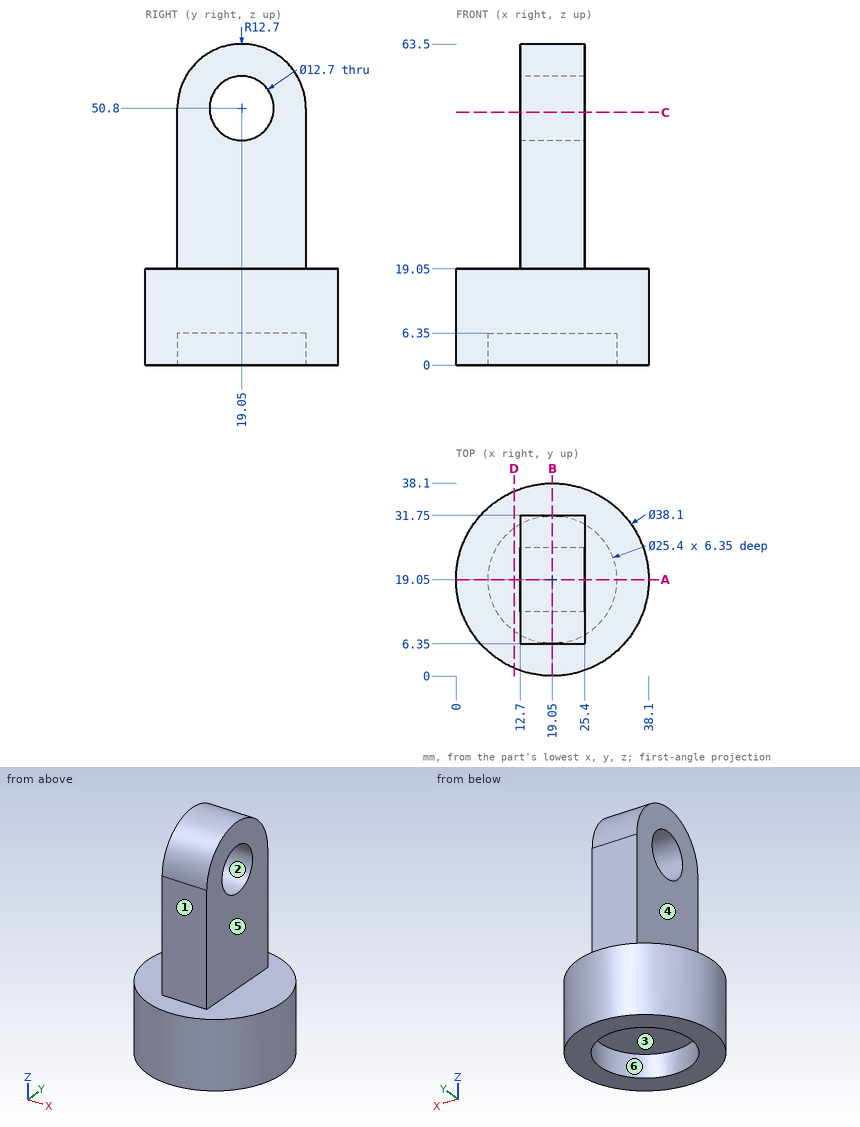
Can you work these out from the drawing? Everything is in mm from the part's minimum corner. A direction names the side the tool comes from. Round coordinates to 2 decimals unless told otherwise and drop trailing zeros. Loops run counter-clockwise (first coordinate to the right, second up) from the corner with the lowest first, then second, coordinate; pieces in that order, holes last. Notation, with made-up numbers: (18.5, -15.75) -> (67.5, -15.75) arc R15 ccw to (67.5, 10.25) -> close; hole circle Ø3 at (45.5, 76). An arc over 180 degrees is marked (long way). One line per question, with ' | ' between items.
(1) If we section it at D-D on x = 11.5: List the corners of the cut face in (y, z) for me.
Model answer:
outline: (1.56, 0) -> (8.84, 0) -> (8.84, 6.35) -> (29.26, 6.35) -> (29.26, 0) -> (36.54, 0) -> (36.54, 19.05) -> (1.56, 19.05) -> close
(2) If I drill on probe 1 along Y at (x, z) = (19.05, 4); probe 2 along Z at (x, y) = (34.5, 30), over which ranges is the centre line in solid material (lowest first)?
Model answer:
probe 1: y = 0 to 6.35, 31.75 to 38.1 | probe 2: z = 0 to 19.05
(3) If we section it at B-B on x = 19.05: List the corners of the cut face in (y, z) for me, and give its area (3 significant figures).
Model answer:
outline: (0, 0) -> (6.35, 0) -> (6.35, 6.35) -> (31.75, 6.35) -> (31.75, 0) -> (38.1, 0) -> (38.1, 19.05) -> (31.75, 19.05) -> (31.75, 50.8) arc R12.7 ccw to (6.35, 50.8) -> (6.35, 19.05) -> (0, 19.05) -> close; hole circle Ø12.7 at (19.05, 50.8) | area: 1,500 mm^2
(4) For the marked faces 4, 5 and 6, which set-ups out of +Z, -Z, +X, -X, +Y, -Y let a thin tool reach every point of the face, with its end or its side?
Model answer:
face 4: +Z, -X, +Y, -Y | face 5: +Z, +X, +Y, -Y | face 6: -Z
(5) If we section it at C-C on z = 50: List the corners of the cut face in (x, y) for me.
Model answer:
outline: (12.7, 6.35) -> (25.4, 6.35) -> (25.4, 12.75) -> (12.7, 12.75) -> close; (12.7, 25.35) -> (25.4, 25.35) -> (25.4, 31.75) -> (12.7, 31.75) -> close
(6) If we section it at A-A on y = 19.05: List the corners of the cut face in (x, z) for me, and give its area (3 significant figures).
Model answer:
outline: (0, 0) -> (6.35, 0) -> (6.35, 6.35) -> (31.75, 6.35) -> (31.75, 0) -> (38.1, 0) -> (38.1, 19.05) -> (25.4, 19.05) -> (25.4, 44.45) -> (12.7, 44.45) -> (12.7, 19.05) -> (0, 19.05) -> close; (12.7, 57.15) -> (25.4, 57.15) -> (25.4, 63.5) -> (12.7, 63.5) -> close | area: 968 mm^2
(7) Thinking about a two-plate mould opening in Z: for the marked faces 1, 2 and 3, which applies, released by +Z, released by -Z, zero draft, split by the parting line, or undercut?
Model answer:
face 1: zero draft | face 2: undercut | face 3: released by -Z
(8) For pin 1 Ø7.5 at (y, z) = (15, 36.5) entering from -X; pin 2 Ø10 at (x, z) = (19.5, 27) entering from -Y; pin 3 Ø12 at (y, z) = (22.5, 45.5) entering from +X, each with a flat end and sliding along its axis, tell me the tip position at first contact or that it passes through.
Model answer:
pin 1: stops at x = 12.7 | pin 2: stops at y = 6.35 | pin 3: stops at x = 25.4
